For this review, take the finished solid that the model builds, in its own axes (mm). A direction names the side the tool comes from. Round coordinates to 2 decimals unless told otherwise and drop trailing zeros. Write each loop counter-clockwise with the first axis right and the second up, starting at its lowest first coordinate (ties: lowest second). Pieces come first, ordered by that corner, then holes.
from build123d import *

# Parameters (mm, degrees)
EXTRUDE_1_DEPTH        = 40
FILLET_1_R             = 6
SHELL_1_T              = -2.5
CUT_EXTRUDE_1_DEPTH    = 2
SKETCH_5_W             = 25
SKETCH_5_H             = 17
CUT_EXTRUDE_4_DEPTH    = 1.5
PATTERN_LINEAR_1_COUNT = 5
PATTERN_LINEAR_1_PITCH = 6
SKETCH_6_R             = 4
EXTRUDE_2_DEPTH        = 32.5
SKETCH_7_R             = 1.25
CUT_EXTRUDE_5_DEPTH    = 12


with BuildPart() as part:
    # 草图1 → 凸台-拉伸1 (new body)
    with BuildSketch(Plane.XY):
        with BuildLine():
            Line((-50, -40), (50, -40))
            ThreePointArc((50, -40), (57.071067812, -37.071067812), (60, -30))
            Line((60, -30), (60, 30))
            ThreePointArc((60, 30), (57.071067812, 37.071067812), (50, 40))
            Line((50, 40), (-50, 40))
            ThreePointArc((-50, 40), (-57.071067812, 37.071067812), (-60, 30))
            Line((-60, 30), (-60, -30))
            ThreePointArc((-60, -30), (-57.071067812, -37.071067812), (-50, -40))
        make_face()
    extrude(amount=EXTRUDE_1_DEPTH)

    # 圆角1
    fillet_1_edges = [part.edges().sort_by_distance(p)[0] for p in [
        (57.071067812, -37.071067812, 40),
        (60, 0, 40),
        (57.071067812, 37.071067812, 40),
        (0, 40, 40),
        (-57.071067812, 37.071067812, 40),
        (-60, 0, 40),
        (-57.071067812, -37.071067812, 40),
        (0, -40, 40),
    ]]
    fillet(fillet_1_edges, radius=FILLET_1_R)

    # 抽壳1
    shell_1_openings = [part.faces().sort_by_distance(p)[0] for p in [
        (0, 0, 0),
    ]]
    offset(amount=SHELL_1_T, openings=shell_1_openings, kind=Kind.INTERSECTION)

    # 草图2 → 切除-拉伸1 (cut)
    with BuildSketch(Plane.XY):
        with BuildLine():
            Line((-50, -45), (50, -45))
            ThreePointArc((50, -45), (60.606601718, -40.606601718), (65, -30))
            Line((65, -30), (65, 30))
            ThreePointArc((65, 30), (60.606601718, 40.606601718), (50, 45))
            Line((50, 45), (-50, 45))
            ThreePointArc((-50, 45), (-60.606601718, 40.606601718), (-65, 30))
            Line((-65, 30), (-65, -30))
            ThreePointArc((-65, -30), (-60.606601718, -40.606601718), (-50, -45))
        make_face()
        with BuildLine():
            Line((-50, -38.8), (50, -38.8))
            ThreePointArc((50, -38.8), (56.222539674, -36.222539674), (58.8, -30))
            Line((58.8, -30), (58.8, 30))
            ThreePointArc((58.8, 30), (56.222539674, 36.222539674), (50, 38.8))
            Line((50, 38.8), (-50, 38.8))
            ThreePointArc((-50, 38.8), (-56.222539674, 36.222539674), (-58.8, 30))
            Line((-58.8, 30), (-58.8, -30))
            ThreePointArc((-58.8, -30), (-56.222539674, -36.222539674), (-50, -38.8))
        make_face(mode=Mode.SUBTRACT)
    extrude(amount=CUT_EXTRUDE_1_DEPTH, mode=Mode.SUBTRACT)

    # 草图5 → 切除-拉伸4 (cut, symmetric)
    with BuildSketch(Plane(origin=(0, -12, 0), x_dir=(1, 0, 0), z_dir=(0, 1, 0))):
        with Locations((52.5, -36.5)):
            Rectangle(SKETCH_5_W, SKETCH_5_H)
    cut_extrude_4 = extrude(amount=CUT_EXTRUDE_4_DEPTH, both=True, mode=Mode.SUBTRACT)

    # 阵列(线性)1: 切除-拉伸4 ×5
    with Locations(*[(0, i * PATTERN_LINEAR_1_PITCH, 0) for i in range(1, PATTERN_LINEAR_1_COUNT)]):
        add(cut_extrude_4, mode=Mode.SUBTRACT)

    # 草图6 → 凸台-拉伸2 (add)
    with BuildSketch(Plane.XY.offset(5)):
        with Locations((45, 25)):
            Circle(SKETCH_6_R)
        with Locations((45, -25)):
            Circle(SKETCH_6_R)
        with Locations((-45, 25)):
            Circle(SKETCH_6_R)
        with Locations((-45, -25)):
            Circle(SKETCH_6_R)
    extrude(amount=EXTRUDE_2_DEPTH)

    # 草图7 → 切除-拉伸5 (cut)
    with BuildSketch(Plane.XY.offset(5)):
        with Locations((45, 25)):
            Circle(SKETCH_7_R)
        with Locations((45, -25)):
            Circle(SKETCH_7_R)
        with Locations((-45, 25)):
            Circle(SKETCH_7_R)
        with Locations((-45, -25)):
            Circle(SKETCH_7_R)
    extrude(amount=CUT_EXTRUDE_5_DEPTH, mode=Mode.SUBTRACT)


solid = part.part
(1) For pin 1 Ø4 at (x, y) = (46, 24) entering from -Z; pin 2 Ø1 at (x, y) = (-47, -16) entering from -Z; pin 3 Ø0.8 at (y, z) = (-5.5, 39) entering from +X, all flat-tipped, find the tip position at first contact; note any pin that passes through.
Geometry check:
pin 1: stops at z = 5
pin 2: stops at z = 37.5
pin 3: stops at x = 40
(2) We need section D-D, the plane x = 38.5. Give the boundary of the cut face in (y, z), and give its area (3 significant figures).
Geometry check:
outline: (-40, 2) - (-38.8, 2) - (-38.8, 0) - (-37.5, 0) - (-37.5, 34) arc R3.5 cw to (-34, 37.5) - (34, 37.5) arc R3.5 cw to (37.5, 34) - (37.5, 0) - (38.8, 0) - (38.8, 2) - (40, 2) - (40, 34) arc R6 ccw to (34, 40) - (-34, 40) arc R6 ccw to (-40, 34) - close
area: 373 mm2
(3) For line 1 along Y through (x, z) = (45, 14.75); line 2 along Y through (x, z) = (0, 11.5); line 3 along X through (y, z) = (16, 14), list the stretches that pass through material, from the lowest coordinate up.
Geometry check:
line 1: y = -40 to -37.5, -29 to -26.25, -23.75 to -21, 21 to 23.75, 26.25 to 29, 37.5 to 40
line 2: y = -40 to -37.5, 37.5 to 40
line 3: x = -60 to -57.5, 57.5 to 60
(4) Mouldability with a two-part tool opening along X and no side actions: class faces 4 (the face through (-1, -37.5, 17)), 5 (the face through (52, -4.5, 38)), 6 (the face through (58.289, -2.979, 38.196)) as pulls with the +X half, pulls with the -X half, needs draft (parallel to the pull), parting line crosses it, or undercut.
Geometry check:
face 4: undercut
face 5: needs draft
face 6: pulls with the +X half
(5) We need section A-A, the plane z = 15. State how many separate pieces and enclosed holes the cut face has, and give its area (3 significant figures).
Geometry check:
separate pieces: 5
enclosed holes: 5
area: 1,120 mm2
(6) For faces 1 (the face through (40, 12, 39)), 2 (the face through (59, 6, 28)), 3 (the face through (-45.521, 28.966, 21.022)), list the 3-axis set-ups (+Z, -Z, +X, -X, +Y, -Y) from which the entire face can be reached by the end or side of a thin tool; tool diameter is ignored.
Geometry check:
face 1: +Z, -Z, +X
face 2: +Z, +X
face 3: -Z
